from build123d import *

# Parameters (mm, degrees)
SKETCH1_W           = 214
SKETCH1_H           = 112
BOSS_EXTRUDE1_DEPTH = 49
SKETCH2_W           = 18.2
SKETCH2_H           = 109.6
CUT_EXTRUDE1_DEPTH  = 41.6
SHELL1_START        = -54.8
SHELL1_DEPTH        = 109.6
SKETCH3_R           = 1.5
CUT_EXTRUDE2_DEPTH  = 10
CUT_EXTRUDE3_START  = -10
SKETCH4_R           = 1.5
CUT_EXTRUDE3_DEPTH  = 10
SKETCH5_W           = 109.6
SKETCH5_H           = 24.5
BOSS_EXTRUDE2_DEPTH = 1.2
SKETCH6_R           = 1.998023928
CUT_EXTRUDE5_DEPTH  = 10
SKETCH7_R           = 1.5
CUT_EXTRUDE6_DEPTH  = 10


# Read off the part's stored shape, not the designer's step: Shell1
with BuildPart() as part:
    # Sketch1 → Boss-Extrude1 (new body)
    with BuildSketch(Plane(origin=(0, 0, 0), x_dir=(1, 0, 0), z_dir=(0, 1, 0))):
        Rectangle(SKETCH1_W, SKETCH1_H)
    extrude(amount=BOSS_EXTRUDE1_DEPTH)

    # Sketch2 → Cut-Extrude1 (cut)
    with BuildSketch(Plane(origin=(0, 49, 0), x_dir=(1, 0, 0), z_dir=(0, 1, 0))):
        with Locations((97.9, 0)):
            Rectangle(SKETCH2_W, SKETCH2_H)
    extrude(amount=-CUT_EXTRUDE1_DEPTH, mode=Mode.SUBTRACT)

    # Shell1 outline → Shell1 (cut)
    with BuildSketch(Plane.XY.offset(SHELL1_START)):
        Polygon((88.8, 6.2), (88.8, 47.8), (-105.8, 47.8), (-105.8, 1.2), (105.8, 1.2), (105.8, 6.2), align=None)
    extrude(amount=SHELL1_DEPTH, mode=Mode.SUBTRACT)

    # Sketch3 → Cut-Extrude2 (cut)
    with BuildSketch(Plane.XY.offset(56)):
        with Locations((75, 11)):
            Circle(SKETCH3_R)
        with Locations((-75, 11)):
            Circle(SKETCH3_R)
    extrude(amount=-CUT_EXTRUDE2_DEPTH, mode=Mode.SUBTRACT)

    # Sketch4 → Cut-Extrude3 (cut)
    with BuildSketch(Plane(origin=(0, 0, -56), x_dir=(-1, 0, 0), z_dir=(0, 0, -1)).offset(CUT_EXTRUDE3_START)):
        with Locations(Location((-75, 11, 0), (0, 0, 180))):
            Circle(SKETCH4_R)
        with Locations((-75, 36)):
            Circle(SKETCH4_R)
        with Locations((75, 36)):
            Circle(SKETCH4_R)
        with Locations(Location((75, 11, 0), (0, 0, 180))):
            Circle(SKETCH4_R)
    extrude(amount=CUT_EXTRUDE3_DEPTH, mode=Mode.SUBTRACT)

    # Sketch5 → Boss-Extrude2 (add)
    with BuildSketch(Plane(origin=(88.8, 0, 0), x_dir=(0, 0, -1), z_dir=(1, 0, 0))):
        with Locations((0, 36.75)):
            Rectangle(SKETCH5_W, SKETCH5_H)
    extrude(amount=BOSS_EXTRUDE2_DEPTH)

    # Sketch6 → Cut-Extrude5 (cut)
    with BuildSketch(Plane(origin=(0, 49, 0), x_dir=(1, 0, 0), z_dir=(0, 1, 0))):
        with Locations(Location((-55.192236422, -23.459739828, 0), (0, 0, 270))):
            Circle(SKETCH6_R)
        with Locations(Location((-62.461489091, -23.807661774, 0), (0, 0, 270))):
            Circle(SKETCH6_R)
        with Locations(Location((-62.809411037, -16.538409104, 0), (0, 0, 270))):
            Circle(SKETCH6_R)
        with Locations(Location((-55.540158368, -16.190487158, 0), (0, 0, 270))):
            Circle(SKETCH6_R)
        with BuildLine():
            ThreePointArc((-68.111702611, -47.500442825), (-58.4348804, -48.96511902), (-48.822553365, -47.124104778))
            ThreePointArc((-48.822553365, -47.124104778), (-47.37733306, -43.943008007), (-50.558429832, -42.497787702))
            ThreePointArc((-50.558429832, -42.497787702), (-58.531267819, -44.024796535), (-66.557600615, -42.809937118))
            ThreePointArc((-66.557600615, -42.809937118), (-69.679904466, -44.378138973), (-68.111702611, -47.500442825))
        make_face()
        with BuildLine():
            ThreePointArc((-87.372467764, -25.85973106), (-83.802503452, -34.97244302), (-77.401974833, -42.376455301))
            ThreePointArc((-77.401974833, -42.376455301), (-73.924454064, -42.037504413), (-74.263404952, -38.559983645))
            ThreePointArc((-74.263404952, -38.559983645), (-79.572252387, -32.418807824), (-82.533319668, -24.860370016))
            ThreePointArc((-82.533319668, -24.860370016), (-85.452574238, -22.940476489), (-87.372467764, -25.85973106))
        make_face()
        with BuildLine():
            ThreePointArc((-78.261444197, 1.640936741), (-84.368302096, -6.007099023), (-87.580100511, -15.252125546))
            ThreePointArc((-87.580100511, -15.252125546), (-85.547800047, -18.09427143), (-82.705654164, -16.061970966))
            ThreePointArc((-82.705654164, -16.061970966), (-80.041663611, -8.393786313), (-74.976398096, -2.050207921))
            ThreePointArc((-74.976398096, -2.050207921), (-74.773348815, 1.437887461), (-78.261444197, 1.640936741))
        make_face()
        with BuildLine():
            ThreePointArc((-49.889655476, 7.500892778), (-59.566477687, 8.965568974), (-69.178804722, 7.124554732))
            ThreePointArc((-69.178804722, 7.124554732), (-70.624025026, 3.94345796), (-67.442928255, 2.498237655))
            ThreePointArc((-67.442928255, 2.498237655), (-59.470090268, 4.025246488), (-51.443757472, 2.810387072))
            ThreePointArc((-51.443757472, 2.810387072), (-48.321453621, 4.378588927), (-49.889655476, 7.500892778))
        make_face()
        with BuildLine():
            ThreePointArc((-30.628890323, -14.139818987), (-34.198854634, -5.027107026), (-40.599383254, 2.376905254))
            ThreePointArc((-40.599383254, 2.376905254), (-44.076904022, 2.037954367), (-43.737953135, -1.439566401))
            ThreePointArc((-43.737953135, -1.439566401), (-38.4291057, -7.580742222), (-35.468038419, -15.139180031))
            ThreePointArc((-35.468038419, -15.139180031), (-32.548783849, -17.059073557), (-30.628890323, -14.139818987))
        make_face()
        with BuildLine():
            ThreePointArc((-39.73991389, -41.640486788), (-33.633055991, -33.992451023), (-30.421257576, -24.7474245))
            ThreePointArc((-30.421257576, -24.7474245), (-32.453558039, -21.905278617), (-35.295703923, -23.93757908))
            ThreePointArc((-35.295703923, -23.93757908), (-37.959694476, -31.605763734), (-43.02495999, -37.949342126))
            ThreePointArc((-43.02495999, -37.949342126), (-43.228009271, -41.437437507), (-39.73991389, -41.640486788))
        make_face()
        with BuildLine():
            ThreePointArc((-59.000823729, -40.866828037), (-53.078604467, -40.008833538), (-47.643378837, -37.505404311))
            ThreePointArc((-47.643378837, -37.505404311), (-46.963644877, -34.314632642), (-50.154416546, -33.634898681))
            ThreePointArc((-50.154416546, -33.634898681), (-54.387958467, -35.584840284), (-59.000823729, -36.253139252))
            ThreePointArc((-59.000823729, -36.253139252), (-61.307668122, -38.559983645), (-59.000823729, -40.866828037))
        make_face()
        with BuildLine():
            ThreePointArc((-77.072828442, -30.432951252), (-73.368673779, -35.13274633), (-68.483027656, -38.588075187))
            ThreePointArc((-68.483027656, -38.588075187), (-65.379871353, -37.58135623), (-66.38659031, -34.478199926))
            ThreePointArc((-66.38659031, -34.478199926), (-70.192060234, -31.786815877), (-73.077256749, -28.126106859))
            ThreePointArc((-73.077256749, -28.126106859), (-76.228464792, -27.281743209), (-77.072828442, -30.432951252))
        make_face()
        with BuildLine():
            ThreePointArc((-77.072828442, -9.56519768), (-79.290893041, -15.122987258), (-79.840472548, -21.081745342))
            ThreePointArc((-79.840472548, -21.081745342), (-77.417050205, -23.265798054), (-75.232997493, -20.842375711))
            ThreePointArc((-75.232997493, -20.842375711), (-74.804925497, -16.201050059), (-73.077256749, -11.872042073))
            ThreePointArc((-73.077256749, -11.872042073), (-73.921620399, -8.72083403), (-77.072828442, -9.56519768))
        make_face()
        with BuildLine():
            ThreePointArc((-59.000823729, 0.868679105), (-64.923042991, 0.010684606), (-70.358268622, -2.492744621))
            ThreePointArc((-70.358268622, -2.492744621), (-71.038002582, -5.68351629), (-67.847230912, -6.36325025))
            ThreePointArc((-67.847230912, -6.36325025), (-63.613688992, -4.413308647), (-59.000823729, -3.74500968))
            ThreePointArc((-59.000823729, -3.74500968), (-56.693979337, -1.438165287), (-59.000823729, 0.868679105))
        make_face()
        with BuildLine():
            ThreePointArc((-40.928819017, -9.56519768), (-44.63297368, -4.865402602), (-49.518619803, -1.410073745))
            ThreePointArc((-49.518619803, -1.410073745), (-52.621776106, -2.416792702), (-51.615057149, -5.519949006))
            ThreePointArc((-51.615057149, -5.519949006), (-47.809587225, -8.211333055), (-44.92439071, -11.872042073))
            ThreePointArc((-44.92439071, -11.872042073), (-41.773182667, -12.716405723), (-40.928819017, -9.56519768))
        make_face()
        with BuildLine():
            ThreePointArc((-40.928819017, -30.432951252), (-38.710754418, -24.875161674), (-38.161174911, -18.91640359))
            ThreePointArc((-38.161174911, -18.91640359), (-40.584597254, -16.732350878), (-42.768649966, -19.155773221))
            ThreePointArc((-42.768649966, -19.155773221), (-43.196721962, -23.797098873), (-44.92439071, -28.126106859))
            ThreePointArc((-44.92439071, -28.126106859), (-44.080027059, -31.277314902), (-40.928819017, -30.432951252))
        make_face()
    extrude(amount=-CUT_EXTRUDE5_DEPTH, mode=Mode.SUBTRACT)

    # Sketch7 → Cut-Extrude6 (cut)
    with BuildSketch(Plane.XZ):
        with Locations(Location((-75, 24, 0), (0, 0, 270))):
            Circle(SKETCH7_R)
        with Locations(Location((75, 24, 0), (0, 0, 270))):
            Circle(SKETCH7_R)
        with Locations(Location((75, -24, 0), (0, 0, 270))):
            Circle(SKETCH7_R)
        with Locations(Location((-75, -24, 0), (0, 0, 270))):
            Circle(SKETCH7_R)
    extrude(amount=-CUT_EXTRUDE6_DEPTH, mode=Mode.SUBTRACT)


solid = part.part
Input: part model. Units: mm. Frame: model coordinates. A direction names the side the tool comes from. Coordinates: 2 decimals unless noted, no trailing zeros. Order: outer loops, then holes, each group sorted by start corner. A loop starts at its lowest first (then second) coordinate and runs counter-clockwise, first axis right, second up. Notation, with made-up numbers: M 54,38 L 97,38 A22 cw 97,67 Z; hole C 71,46 d9. An arc over 180 degrees is marked long. Answer as CSV lines item,"result".
1. Section C-C (z = -32.5). Return the cut outline in (x, y).
Reported:
outline,"M -107,0 L 107,0 L 107,7.4 L 88.8,7.4 L 88.8,6.2 L 105.8,6.2 L 105.8,1.2 L -105.8,1.2 L -105.8,47.8 L 88.8,47.8 L 88.8,24.5 L 90,24.5 L 90,49 L -107,49 Z"
2. First-contact query: P1, Ø2.5, axis at x = -75, y = 11, coming from the +Z side; P2, Ø19.5, axis at y = 41, z = 16.5, coming from the +X side; P3, Ø2.5, axis at x = 75, z = 24, coming from the -Y side; P4, Ø2.5, axis at x = -75, y = 36, coming from the -Z side. Flat tips, straight axial feed; report the tip coordinate or a pass-through.
Reported:
P1,"through"
P2,"x = 90"
P3,"y = 47.8"
P4,"z = 54.8"
3. Material intervals for line 1 (Z direction, x = 71, y = 25); line 2 (Z direction, x = -75, y = 0.4); line 3 (Y direction, x = 24, z = -22), sorted ascending. Write a range as from..to.
Reported:
line 1,"-56..-54.8, 54.8..56"
line 2,"-56..-25.5, -22.5..22.5, 25.5..56"
line 3,"0..1.2, 47.8..49"
4. Section A-A (x = -28). Return the cut outline in (y, z).
Reported:
outline,"M 0,-56 L 49,-56 L 49,56 L 0,56 Z; hole M 1.2,-54.8 L 47.8,-54.8 L 47.8,54.8 L 1.2,54.8 Z"
5. Access query for faces 1 (the flat face through (-1, 24, -56)), 2 (the flat face through (-1, 1.2, -1)), 3 (the cylindrical face through (-38.49, 48.41, 7.48)), 4 (the flat face through (90, 37, 1)). Directions: +Z, -Z, +X, -X, +Y, -Y. A direction counts if a zero-diameter tool reaches every point of the face in a straight line with its end or side. Return the directions, or none.
Reported:
face 1,"-Z, +X, -X, +Y, -Y"
face 2,"none"
face 3,"+Y"
face 4,"+X, +Y"
6. Section D-D (y = 20.5). Return the cut outline in (x, z).
Reported:
outline,"M -107,-56 L 107,-56 L 107,-54.8 L -105.8,-54.8 L -105.8,54.8 L 107,54.8 L 107,56 L -107,56 Z"
7. Pull-direction query (Y, two-part tool) for faces 5 (the cylindrical face through (-73.43, 48.408, 35.075)), 6 (the flat face through (-1, 0, -1)), 7 (the flat face through (-105.8, 25, -1)); classes: released by +Y, released by -Y, zero draft, split by the parting line, or undercut.
Reported:
face 5,"zero draft"
face 6,"released by -Y"
face 7,"undercut"
8. Section B-B (y = 43). Return the cut outline in (x, z).
Reported:
outline,"M -107,-56 L 107,-56 L 107,-54.8 L 90,-54.8 L 90,54.8 L 107,54.8 L 107,56 L -107,56 Z; hole M -105.8,-54.8 L 88.8,-54.8 L 88.8,54.8 L -105.8,54.8 Z"
